Verification items for the finished model (mm, model axes). A direction names the side the tool comes from. Round coordinates to 2 decimals unless told otherwise and drop trailing zeros. Loops run counter-clockwise (first coordinate to the right, second up) from the corner with the lowest first, then second, coordinate; pieces in that order, holes last. Notation, with made-up numbers: (9.5, -39.5) -> (44.5, -39.5) arc R18 ccw to (44.5, -30.5) -> close; hole circle Ø8 at (-12, 55.25). An arc over 180 degrees is marked (long way). Use a Markdown table: item, result. Add a question column.
```python
from build123d import *

# Parameters (mm, degrees)
F1_DEPTH = 25.4
F3_W     = 130.528664
F3_H     = 12.7
F4_DEPTH = 25.4
F6_D     = 20.32


with BuildPart() as f1:
    # F0 (on Front) → F1 (new body)
    with BuildSketch(Plane.XZ):
        with BuildLine():
            Line((-63.120894, 12.7), (-63.120894, 0))
            Line((-63.120894, 0), (49.977216, 0))
            Line((49.977216, 0), (67.445484, 0))
            Line((67.445484, 0), (67.445484, 47.014621))
            ThreePointArc((67.445484, 47.014621), (49.977216, 53.975), (32.508948, 47.014621))
            Line((32.508948, 47.014621), (-63.120894, 12.7))
        make_face()
        with BuildLine():
            ThreePointArc((61.089716, 28.575), (57.83494, 20.717276), (49.977216, 17.4625))
            ThreePointArc((49.977216, 17.4625), (42.119492, 36.432724), (61.089716, 28.575))
        make_face(mode=Mode.SUBTRACT)
    extrude(amount=F1_DEPTH)

    # F3 (on face) → F4 (join)
    with BuildSketch(Plane.XZ.offset(25.4)):
        with Locations((2.143438, 6.35)):
            Rectangle(F3_W, F3_H)
    extrude(amount=F4_DEPTH)

    # F6 (through all)
    with Locations(Plane.XY.offset(12.7)):
        with Locations((-25.020894, -37.777487), (29.30777, -38.479097)):
            Hole(F6_D / 2)


solid = f1.part
```
1) Sectioned sample at C-C on x = 56. Enter the section's corners in (y, z), then the cut area to 3 significant figures.
2) Access from +Z, -Z, +X, -X, +Y, -Y to the whole of each face (thin tool, end or side, straight path). Record for faces 4 (the face through (1, -38, 12.7)), 5 (the face through (19.923, -42.37, 6.261)).
3) Release check for a two-part mould opening along X. For faces 1 (the face through (50.247, -12.522, 53.974)), 2 (the face through (-23.698, -27.704, 6.261)), 3 (the face through (-63.121, -25, 6)) record: released by +X, released by -X, zero draft, split by the parting line, or undercut.
4) Sectioned sample at B-B on z = 23.5. Enter the section's corners in (x, y), then the cut area to 3 significant figures.
5) Sectioned sample at A-A on y = -9.5. Enter the section's corners in (x, z) (1 decimal).
6) Sectioned sample at D-D on y = -41. Enter the section's corners in (x, z).
7) Go/stop test with flat-tipped pins: pin 1 (16 mm diameter, centred on x = -19, z = 35, fed in from -Y); pin 2 (8 mm diameter, centred on x = -12, y = -41, fed in from +Z); pin 3 (14 mm diameter, centred on y = -38.5, z = 5, fed in from +X). Record where each tip stops, or that it passes through.
8) Thickness scan on line 1 (X direction, y = -37, z = 11.5); line 2 (Y direction, x = 40, z = 44); line 3 (Y direction, x = -17, z = 9). Record the ranges inside material, lowest first.
Geometry results:
| question | item | result |
|---|---|---|
| 1 | outline | (-50.8, 0) -> (0, 0) -> (0, 19.24) -> (-25.4, 19.24) -> (-25.4, 12.7) -> (-50.8, 12.7) -> close; (-25.4, 37.91) -> (0, 37.91) -> (0, 53.25) -> (-25.4, 53.25) -> close |
| 1 | area | 1,200 mm^2 |
| 2 | face 4 | +Z, +X, -X, -Y |
| 2 | face 5 | +Z, -Z |
| 3 | face 1 | split by the parting line |
| 3 | face 2 | undercut |
| 3 | face 3 | released by -X |
| 4 | outline | (-33.02, -25.4) -> (40.09, -25.4) -> (40.09, 0) -> (-33.02, 0) -> close; (59.86, -25.4) -> (67.45, -25.4) -> (67.45, 0) -> (59.86, 0) -> close |
| 4 | area | 2,050 mm^2 |
| 5 | outline | (-63.1, 0) -> (67.4, 0) -> (67.4, 47) arc R25.4 ccw to (32.5, 47) -> (-63.1, 12.7) -> close; hole circle Ø22.2 at (50, 28.6) |
| 6 | outline | (-63.12, 0) -> (-34.66, 0) -> (-34.66, 12.7) -> (-63.12, 12.7) -> close; (-15.39, 0) -> (19.47, 0) -> (19.47, 12.7) -> (-15.39, 12.7) -> close; (39.15, 0) -> (67.41, 0) -> (67.41, 12.7) -> (39.15, 12.7) -> close |
| 7 | pin 1 | y = -25.4 |
| 7 | pin 2 | z = 12.7 |
| 7 | pin 3 | x = 67.41 |
| 8 | line 1 | -63.12 to -35.15, -14.89 to 19.26, 39.36 to 67.41 |
| 8 | line 2 | -25.4 to 0 |
| 8 | line 3 | -50.8 to -44.01, -31.54 to 0 |
